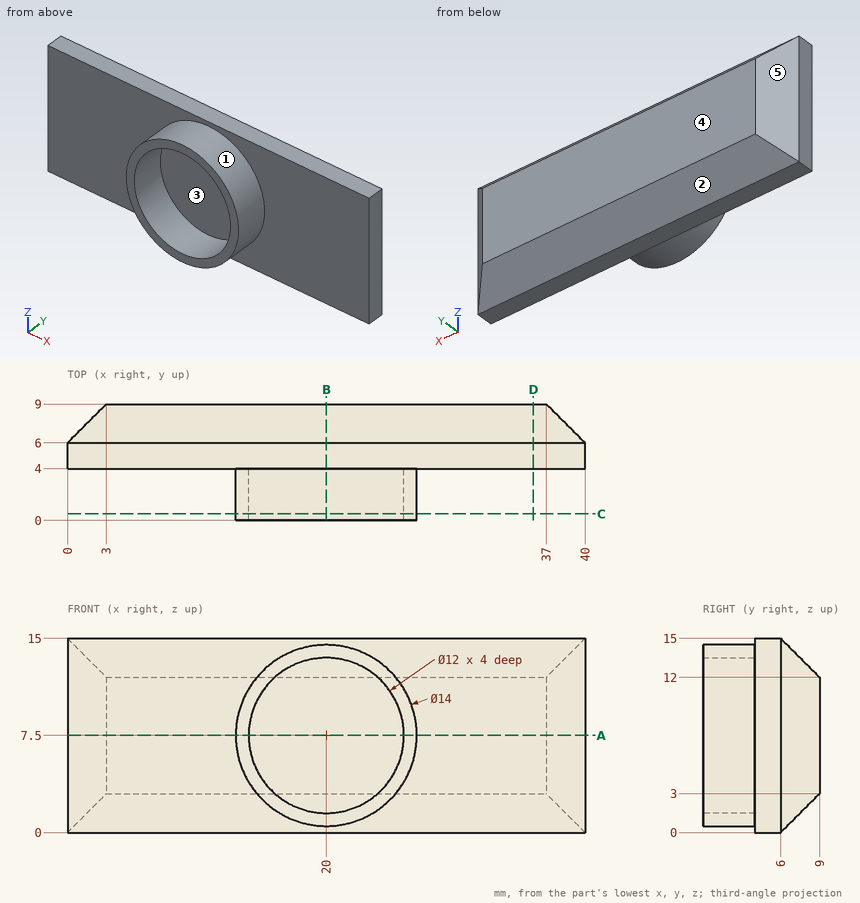
Can you work these out from the drawing? Everything is in mm from the part's minimum corner. A direction names the side the tool comes from. Round coordinates to 2 decimals unless told otherwise and drop trailing zeros. Write each loop counter-clockwise with the first axis right and the second up, starting at its lowest first coordinate (ties: lowest second). Pieces come first, ordered by that corner, then holes. Notation, with made-up numbers: (-30, -7.5) - (-16, -7.5) arc R33 ccw to (-16, 23.5) - close; hole circle Ø6 at (-35.5, 18.25). An arc over 180 degrees is marked (long way). Put each result on its own line as item: value. Start each with the question number.
(1) I want a section at A-A, the plane z = 7.5. Please give me the cut outline in (x, y).
(2) Thinking about a two-plate mould opening in X: for the marked faces 3, 4 and 5, which applies, released by +X, released by -X, zero draft, split by the parting line, or undercut?
(3) I need wall thicknesses on probe 1 along X at (y, z) = (2.8, 7.5); probe 2 along Y at (x, z) = (35, 9.5); probe 3 along Z at (x, y) = (19.5, 3.25). Which ranges of each line are inside material? Lowest first, please.
(4) For the marked faces 1 and 2, which set-ups out of +Z, -Z, +X, -X, +Y, -Y let a thin tool reach every point of the face, with its end or its side?
(5) I want a section at C-C, the plane y = 0.5. Please give me the cut outline in (x, z), plus the area to 3 significant figures.
(6) I want a section at D-D, the plane x = 36. Please give me the cut outline in (y, z).
(7) Will this pin go through, and if not, where does the flat tip stop? pin 1 (3 mm diameter, centred on x = 7, z = 10, fed in from -Y).
(8) I want a section at B-B, the plane x = 20. Please give me the cut outline in (y, z), plus the area to 3 significant figures.
Here are the results:
1. outline: (0, 4) - (13, 4) - (13, 0) - (14, 0) - (14, 4) - (26, 4) - (26, 0) - (27, 0) - (27, 4) - (40, 4) - (40, 6) - (37, 9) - (3, 9) - (0, 6) - close
2. face 3: undercut
2. face 4: zero draft
2. face 5: released by -X
3. probe 1: x = 13 to 14, 26 to 27
3. probe 2: y = 4 to 9
3. probe 3: z = 0.52 to 1.52, 13.48 to 14.48
4. face 1: -Y
4. face 2: -Z, +X, -X, +Y
5. outline: circle Ø14 at (20, 7.5); hole circle Ø12 at (20, 7.5)
5. area: 40.8 mm^2
6. outline: (4, 0) - (6, 0) - (9, 3) - (9, 12) - (6, 15) - (4, 15) - close
7. pin 1: stops at y = 4
8. outline: (0, 0.5) - (4, 0.5) - (4, 0) - (6, 0) - (9, 3) - (9, 12) - (6, 15) - (4, 15) - (4, 14.5) - (0, 14.5) - (0, 13.5) - (4, 13.5) - (4, 1.5) - (0, 1.5) - close
8. area: 74.0 mm^2
